from build123d import *

# Parameters (mm, degrees)
F0_R     = 14
F0_R_2   = 12
F1_DEPTH = 16
F3_DEPTH = 2.5
F4_W     = 28
F4_H     = 28
F5_DEPTH = 5
F6_W     = 5
F6_H     = 0.75
F6_W_2   = 0.375
F6_H_2   = 2.5
F7_DEPTH = 5.001


with BuildPart() as f1:
    # F0 (on Top) → F1 (new body)
    with BuildSketch(Plane.XY):
        Circle(F0_R)
        Circle(F0_R_2, mode=Mode.SUBTRACT)
    extrude(amount=F1_DEPTH)

    # F2 (on Top) → F3 (join)
    with BuildSketch(Plane.XY):
        with BuildLine():
            Line((-11.2159206042, 0.875), (-11.968056442, 0.875))
            ThreePointArc((-11.968056442, 0.875), (-12, 0), (-11.968056442, -0.875))
            Line((-11.968056442, -0.875), (-11.2159206042, -0.875))
            ThreePointArc((-11.2159206042, -0.875), (-11.25, 0), (-11.2159206042, 0.875))
        make_face()
        with BuildLine():
            ThreePointArc((11.968056442, -0.875), (12, 0), (11.968056442, 0.875))
            Line((11.968056442, 0.875), (11.2159206042, 0.875))
            ThreePointArc((11.2159206042, 0.875), (11.25, 0), (11.2159206042, -0.875))
            Line((11.2159206042, -0.875), (11.968056442, -0.875))
        make_face()
    extrude(amount=F3_DEPTH)

    # F4 (on face) → F5 (join)
    with BuildSketch(Plane.XY.offset(16)):
        Rectangle(F4_W, F4_H)
    extrude(amount=F5_DEPTH)

    # F6 (on face) → F7 (cut, through all)
    with BuildSketch(Plane(origin=(0, 0, 16), x_dir=(1, 0, 0), z_dir=(0, 0, -1))):
        with Locations((0, -2.8625)):
            Rectangle(F6_W, F6_H)
        with Locations((0.1875, -7.9375)):
            Rectangle(F6_W_2, F6_H_2)
        with Locations((-0.1875, -7.9375)):
            Rectangle(F6_W_2, F6_H_2)
        Polygon((5.6040448878, 3.6685095264), (5.7915448878, 3.34375), (7.9566083973, 4.59375), (7.7691083973, 4.9185095264), align=None)
        Polygon((7.9566083973, 4.59375), (5.7915448878, 3.34375), (5.9790448878, 3.0189904736), (8.1441083973, 4.2689904736), align=None)
        Polygon((-5.9790448878, 3.0189904736), (-5.7915448878, 3.34375), (-7.9566083973, 4.59375), (-8.1441083973, 4.2689904736), align=None)
        Polygon((-7.9566083973, 4.59375), (-5.7915448878, 3.34375), (-5.6040448878, 3.6685095264), (-7.7691083973, 4.9185095264), align=None)
    extrude(amount=-F7_DEPTH, mode=Mode.SUBTRACT)


solid = f1.part
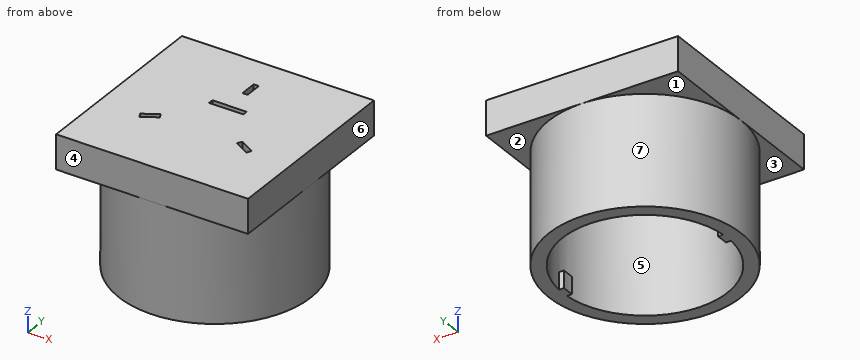
Input: part model. Units: mm. Frame: model coordinates. Face numbers are marked on the shaded views. A direction names the side the tool comes from. Give positions to 0.01 mm unless a question says otherwise; leave off trailing zeros. Loops run counter-clockwise (first coordinate to the right, second up) from the corner with the lowest first, then second, coordinate; pieces in that order, holes last. Notation, with made-up numbers: (15.25, 13.25) -> (25.25, 13.25) arc R33 ccw to (25.25, 42.25) -> close; hole circle Ø2 at (79.25, -36). An arc over 180 degrees is marked (long way). Answer as a JSON object with one key per item and string values. Group by question number.
Item 1: Pull-direction query (Y, two-part tool) for the marked faces 4, 5, 6 and 7; classes: released by +Y, released by -Y, zero draft, split by the parting line, or undercut.
Item 2: Pin query (flat end, axial travel): P1, Ø5, axis at x = 6.5, y = -4.5, coming from the -Z side; P2, Ø3, axis at x = -8.5, z = 8, coming from the -Y side; P3, Ø0.6, axis at x = -11.5, z = 0.5, coming from the -Y side. Return the tip coordinate at first contact, or that it passes through.
Item 3: Cut plane C-C, the plane z = 6.75. Return the cut outline in (x, y), and give its area (3 significant figures).
Item 4: Reachability of the marked faces 1, 2 and 3 from +Z, -Z, +X, -X, +Y, -Y: full face, straight path, thin tool, end or side. Return the list, or none.
Item 5: Cut plane D-D, the plane x = 9.5. Return the cut outline in (y, z).
Item 6: Line query: probe 1 along X at (y, z) = (-4, 19.75); probe 2 along Y at (x, z) = (0, 11.25); probe 3 along Z at (x, y) = (0.25, -3.25). Output: solid intervals per line, ascending.
Checks:
{
 "1": {"face 4": "released by -Y", "face 5": "undercut", "face 6": "zero draft", "face 7": "split by the parting line"},
 "2": {"P1": "stops at z = 16", "P2": "stops at y = -12.12", "P3": "stops at y = -8.4"},
 "3": {"outline": "circle Ø28 at (0, 0); hole circle Ø24 at (0, 0)", "area": "163 mm²"},
 "4": {"face 1": "-Z, -X, +Y", "face 2": "-Z, +X, +Y", "face 3": "-Z, -X, -Y"},
 "5": {"outline": "(-14, 16) -> (-10.28, 16) -> (-10.28, 0) -> (-7.33, 0) -> (-7.33, 16) -> (7.33, 16) -> (7.33, 0) -> (10.28, 0) -> (10.28, 16) -> (14, 16) -> (14, 21) -> (-14, 21) -> close"},
 "6": {"probe 1": "x = -14 to -7.68, -6.18 to 6.18, 7.68 to 14", "probe 2": "y = -14 to -12, 12 to 14", "probe 3": "z = 16 to 21"}
}
